```python
from build123d import *

# Parameters (mm, degrees)
F0_W          = 10
F0_H          = 43.1
F0_R          = 1.55
F1_DEPTH      = 10
F0_H_2        = 31.9
F2_DEPTH      = 10
F2_DEPTH_BACK = 6
F0_H_3        = 10
F3_DEPTH      = 30
F3_DEPTH_BACK = 10
F4_R          = 1.55
F5_DEPTH      = 15
F6_R          = 1
F7_R          = 1.55
F8_DEPTH      = 3
F9_R          = 2.5
F10_DEPTH     = 3


with BuildPart() as f1:
    # F0 (on Top) → F1 (new body)
    with BuildSketch(Plane.XY):
        with Locations((-5, 21.55)):
            Rectangle(F0_W, F0_H)
        with Locations((-5, 5)):
            Circle(F0_R, mode=Mode.SUBTRACT)
        with Locations((-5, 38.1)):
            Circle(F0_R, mode=Mode.SUBTRACT)
    extrude(amount=F1_DEPTH)

    # F0 (on Top) → F2 (join, two sides)
    with BuildSketch(Plane.XY) as f2_sk:
        with Locations((-5, 59.05)):
            Rectangle(F0_W, F0_H_2)
    extrude(amount=F2_DEPTH)
    extrude(f2_sk.sketch, amount=-F2_DEPTH_BACK)

    # F0 (on Top) → F3 (join, two sides)
    with BuildSketch(Plane.XY) as f3_sk:
        with Locations((-5, 80)):
            Rectangle(F0_W, F0_H_3)
    extrude(amount=-F3_DEPTH)
    extrude(f3_sk.sketch, amount=F3_DEPTH_BACK)

    # F4 (on face) → F5 (cut)
    with BuildSketch(Plane(origin=(0, 85, 0), x_dir=(-1, 0, 0), z_dir=(0, 1, 0))):
        with Locations((5, -25)):
            Circle(F4_R)
        with Locations((5, -10)):
            Circle(F4_R)
    extrude(amount=-F5_DEPTH, mode=Mode.SUBTRACT)

    # F6
    f6_edges = [f1.edges().sort_by_distance(p)[0] for p in [
        (-10, 42.5, 10),
        (0, 42.5, 10),
        (-5, 85, 10),
        (-10, 75, -18),
        (-5, 75, -30),
        (0, 80, -30),
        (-10, 80, -30),
        (-10, 0, 5),
        (0, 0, 5),
        (-5, 0, 10),
        (0, 75, -18),
    ]]
    fillet(f6_edges, radius=F6_R)

    # F7 (on face) → F8 (cut)
    with BuildSketch(Plane.XZ.offset(-75)):
        Polygon((-2.25, -11.5877132403), (-2.25, -8.4122867597), (-5, -6.8245735195), (-7.75, -8.4122867597), (-7.75, -11.5877132403), (-5, -13.1754264805), align=None)
        with Locations((-5, -10)):
            Circle(F7_R, mode=Mode.SUBTRACT)
        Polygon((-2.25, -26.5877132403), (-2.25, -23.4122867597), (-5, -21.8245735195), (-7.75, -23.4122867597), (-7.75, -26.5877132403), (-5, -28.1754264805), align=None)
        with Locations((-5, -25)):
            Circle(F7_R, mode=Mode.SUBTRACT)
    extrude(amount=-F8_DEPTH, mode=Mode.SUBTRACT)

    # F9 (on face) → F10 (cut)
    with BuildSketch(Plane.XY.offset(10)):
        with Locations((-5, 38.1)):
            Circle(F9_R)
        with Locations((-5, 5)):
            Circle(F9_R)
    extrude(amount=-F10_DEPTH, mode=Mode.SUBTRACT)


solid = f1.part
```
The listing builds one solid part. Answer for the finished solid, in the listing's coordinates (mm). A direction names the side the tool comes from. Give positions to 0.01 mm unless a question says otherwise; leave off trailing zeros. Order: outer loops, then holes, each group sorted by start corner. A loop starts at its lowest first (then second) coordinate and runs counter-clockwise, first axis right, second up. Notation, with made-up numbers: (78.25, 20) -> (82.25, 20) arc R11 ccw to (82.25, 39) -> close; hole circle Ø8 at (9.25, -19.5). An arc over 180 degrees is marked (long way). Answer as CSV lines item,"result". Start each with the question number.
Q1. Given pin 1 (6 mm diameter, centred on x = -4.5, z = -11, fed in from -Y); pin 2 (4 mm diameter, centred on x = -5, y = 38.1, fed in from +Z); pin 3 (4 mm diameter, centred on x = -5, y = 38.1, fed in from -Z), each flat-ended and moving along its own axis, determine where each tip first touches the part or whether it passes through.
Q2. A cutting plane is placed at A-A (z = -25). Determine the outline of the cut face in (x, y).
Q3. Determine the mould class of faces 1 (the flat face through (-10, 55, 0)), 2 (the flat face through (-3.8, 78, -26.4)), 3 (the flat face through (-3, 5, 7)) for opening direction Z: pulls with the +Z half, pulls with the -Z half, needs draft (parallel to the pull), parting line crosses it, or undercut.
Q4. Find the intervals of material crossed by L1, parallel to Y at x = -5, z = 4.75; L2, parallel to X at y = 80.75, z = -25; L3, parallel to Z at x = -7.5, y = 75.5, in increasing order.
Q5. A cutting plane is placed at D-D (y = 10). Determine the outline of the cut face in (x, z), then the cut area to 3 significant figures.
Q6. Which of the six approach directions +Z, -Z, +X, -X, +Y, -Y give full straight-line access (tool end or side, diameter ignored) to faces 4 (the flat face through (-6.394, 76.479, -27.37)), 5 (the cylindrical face through (-6.55, 5.07, 3.45)), 6 (the flat face through (-5, 75, -17))?
Q7. A cutting plane is placed at C-C (z = 6). Determine the outline of the cut face in (x, y), then the cut area to 3 significant figures.
Q8. A cutting plane is placed at B-B (y = 38.1). Determine the outline of the cut face in (x, z), then the cut area to 3 significant figures.
Results found:
1,pin 1,"y = 75"
1,pin 2,"z = 7"
1,pin 3,"z = 0"
2,outline,"(-10, 76) arc R1 ccw to (-9, 75) -> (-7.75, 75) -> (-7.75, 78) -> (-6.55, 78) -> (-6.55, 85) -> (-10, 85) -> close; (-3.45, 78) -> (-2.25, 78) -> (-2.25, 75) -> (-1, 75) arc R1 ccw to (0, 76) -> (0, 85) -> (-3.45, 85) -> close"
3,face 1,"needs draft"
3,face 2,"undercut"
3,face 3,"pulls with the +Z half"
4,L1,"0 to 3.45, 6.55 to 36.55, 39.65 to 85"
4,L2,"-10 to -6.55, -3.45 to 0"
4,L3,"-29.87 to -26.73, -23.27 to -11.73, -8.27 to 10"
5,outline,"(-10, 0) -> (0, 0) -> (0, 9) arc R1 ccw to (-1, 10) -> (-9, 10) arc R1 ccw to (-10, 9) -> close"
5,area,"99.6 mm2"
6,face 4,"-Y"
6,face 5,"+Z, -Z"
6,face 6,"-Z, +X, -X, -Y"
7,outline,"(-10, 1) arc R1 ccw to (-9, 0) -> (-1, 0) arc R1 ccw to (0, 1) -> (0, 85) -> (-10, 85) -> close; hole circle Ø3.1 at (-5, 5); hole circle Ø3.1 at (-5, 38.1)"
7,area,"834 mm2"
8,outline,"(-10, 0) -> (-6.55, 0) -> (-6.55, 7) -> (-7.5, 7) -> (-7.5, 10) -> (-9, 10) arc R1 ccw to (-10, 9) -> close; (-3.45, 0) -> (0, 0) -> (0, 9) arc R1 ccw to (-1, 10) -> (-2.5, 10) -> (-2.5, 7) -> (-3.45, 7) -> close"
8,area,"62.9 mm2"
